The listing builds one solid part. Answer for the finished solid, in the listing's coordinates (mm). A direction names the side the tool comes from. Round coordinates to 2 decimals unless told otherwise and drop trailing zeros. Loops run counter-clockwise (first coordinate to the right, second up) from the corner with the lowest first, then second, coordinate; pieces in that order, holes last. Notation, with made-up numbers: (77.25, 78) -> (87.25, 78) arc R17 ccw to (87.25, 99) -> close; hole circle Ø6 at (-14.5, 47). An arc over 180 degrees is marked (long way). One line per question, with ' | ' between items.
Autodesk Inventor part; units mm, degrees
ref_plane "Work Plane6" through (-3.7586, 19.05, -25.4) normal (-0.342, 0.9397, 0) x (0, 0, 1)
ref_plane "YZ Plane" through (0, 0, 0) normal (1, 0, 0) x (0, 1, 0)
ref_plane "XZ Plane" through (0, 0, 0) normal (0, 1, 0) x (-1, 0, 0)
sketch "Sketch1" plane through (0, 0, 0) normal (0, 1, 0) x (-1, 0, 0)
  line L0 (0, 0) -> (-12.7, 0)
  line L1 (-12.7, 0) -> (-12.7, -25.4)
  line L2 (-12.7, -25.4) -> (0, -25.4)
  line L3 (0, -25.4) -> (0, 0)
  line L4 (0, -12.7) -> (-12.7, -12.7) construction
  line L5 (-3.175, -25.4) -> (-3.175, 0)
  line L6 (-3.175, -20.8831) -> (0, -19.05)
  line L7 (-3.175, -4.5169) -> (0, -6.35)
  line L8 (-9.525, -25.4) -> (-9.525, 0)
  point P0 (-3.175, -12.7)
  point P1 (0, -6.35)
  dimension "d0" = 12.7
  dimension "d7" = 25.4
  dimension "d34" = 3.175
  dimension "d35" = 60
  dimension "d36" = 12.7
  dimension "d57" = 3.175
sketch "Sketch8" plane through (0, 0, 0) normal (0, 0, 1) x (1, 0, 0)
  line L0 (0, 0) -> (-6.9336, 19.05)
  line L1 (0, 0) -> (20.2726, 0) construction
  dimension "d53" = 110
  dimension "d54" = 19.05
sweep "Sweep3" add profiles "Sketch1" path "Sketch8" contours L3 L7 L5 L0 | L5 L2 L8 L0 | L8 L2 L1 L0 | L3 L2 L5 L6
extrude "Extrusion3" add sketch "Sketch1" along normal blind 6.35 contours L8 L2 L1 L0
ref_plane "Work Plane6" through (-3.7586, 19.05, -25.4) normal (-0.342, 0.9397, 0) x (0, 0, 1)
sketch "Sketch9" plane through (-3.7586, 19.05, -25.4) normal (-0.342, 0.9397, 0) x (0, 0, 1)
  line L0 (4.5169, 0) -> (20.8831, 0) construction
  point P0 (12.7, 0)
hole "Hole4" at (-3.7586, 19.05, -12.7) direction (0.342, -0.9397, 0) diameter 6.7564 depth 12.7 tip angle 118
equation "\"slopeAngle\" = 70deg"
properties material "Steel, Alloy"
Q1. Find the intervals of material crossed by line 1 (Y direction, x = 11.75, z = -5); line 2 (Z direction, x = -4.75, y = 14.5); line 3 (Z direction, x = 1.5, y = 10.75), in increasing order. Write a range as from..to.
Numbers:
line 1: 0..6.35 | line 2: -25.4..-19.35, -6.05..0 | line 3: -25.4..-15.34, -10.06..0
Q2. For a pull along Z with two mould halves and no side action, classify faces 4 (the face through (3, 10, -25.4)), 5 (the face through (-1.95, 9.658, -19.954)), 6 (the face through (6, 0, -13)) as pulls with the +Z half, pulls with the -Z half, needs draft (parallel to the pull), parting line crosses it, or undercut.
Numbers:
face 4: pulls with the -Z half | face 5: undercut | face 6: needs draft
Q3. A cutting plane is placed at A-A on x = -5.5. Give the vertices of the cut face in (y, z).
Numbers:
outline: (15.11, -25.4) -> (19.05, -25.4) -> (19.05, -19.88) -> (15.11, -19.05) -> close; (15.11, -6.35) -> (19.05, -5.52) -> (19.05, 0) -> (15.11, 0) -> close
Q4. A cutting plane is placed at C-C on y = 1.75. Give the vertices of the cut face in (x, z), plus the area to 3 significant figures.
Numbers:
outline: (-0.64, -25.4) -> (12.7, -25.4) -> (12.7, 0) -> (-0.64, 0) -> (-0.64, -6.35) -> (2.54, -4.52) -> (2.54, -20.88) -> (-0.64, -19.05) -> close | area: 293 mm^2
Q5. For faces 1 (the face through (-1.833, 9.658, -5.379)), 2 (the face through (12, 6.35, -13)), 3 (the face through (3, 10, 0)), determine the directions among +Z, -Z, +X, -X, +Y, -Y from which every point of the face is accessible in a straight line to the end or side of a thin tool.
Numbers:
face 1: none | face 2: +Z, -Z, +X, +Y | face 3: +Z, +X, -X, +Y, -Y
Q6. A cutting plane is placed at D-D on x = 9.5. Give the vertices of the cut face in (y, z).
Numbers:
outline: (0, -25.4) -> (8.79, -25.4) -> (8.79, 0) -> (0, 0) -> close
Q7. A cutting plane is placed at B-B on z = -7.25. Give the vertices of the cut face in (x, y) (3 decimals), plus the area to 3 significant figures.
Numbers:
outline: (-3.759, 19.05) -> (3.175, 0) -> (12.7, 0) -> (12.7, 6.35) -> (10.389, 6.35) -> (5.766, 19.05) -> close | area: 189 mm^2
Q8. Given pin 1 Ø2 at (x, z) = (-2, -13.5) entering from +Y; pin 2 Ø1.2 at (x, z) = (11.5, -9) entering from +Y, each flat-ended and moving along its own axis, determine where each tip first touches the part or whether it passes through.
Numbers:
pin 1: through | pin 2: y = 6.35
